```python
from build123d import *

# Parameters (mm, degrees)
SKETCH1_R           = 174.85
SKETCH1_R_2         = 3.556
SKETCH1_R_3         = 162.15
BOSS_EXTRUDE1_DEPTH = 3.175


with BuildPart() as part:
    # Sketch1 → Boss-Extrude1 (new body)
    with BuildSketch(Plane(origin=(0, 0, 0), x_dir=(1, 0, 0), z_dir=(0, 1, 0))):
        Circle(SKETCH1_R)
        with Locations((0, 168.5)):
            Circle(SKETCH1_R_2, mode=Mode.SUBTRACT)
        with Locations((145.925280538, 84.25)):
            Circle(SKETCH1_R_2, mode=Mode.SUBTRACT)
        with Locations((145.925280538, -84.25)):
            Circle(SKETCH1_R_2, mode=Mode.SUBTRACT)
        with Locations((0, -168.5)):
            Circle(SKETCH1_R_2, mode=Mode.SUBTRACT)
        with Locations((-145.925280538, -84.25)):
            Circle(SKETCH1_R_2, mode=Mode.SUBTRACT)
        with Locations((-145.925280538, 84.25)):
            Circle(SKETCH1_R_2, mode=Mode.SUBTRACT)
        Circle(SKETCH1_R_3, mode=Mode.SUBTRACT)
    extrude(amount=BOSS_EXTRUDE1_DEPTH)


solid = part.part
```
For this review, take the finished solid that the model builds, in its own axes (mm). Round coordinates to 2 decimals unless told otherwise and drop trailing zeros. Order: outer loops, then holes, each group sorted by start corner. A loop starts at its lowest first (then second) coordinate and runs counter-clockwise, first axis right, second up.
Q1. We need section C-C, the plane y = 2.35. Give the boundary of the cut face in (x, z).
Findings below:
outline: circle Ø349.7 at (0, 0); hole circle Ø324.3 at (0, 0); hole circle Ø7.11 at (-145.93, -84.25); hole circle Ø7.11 at (-145.93, 84.25); hole circle Ø7.11 at (0, -168.5); hole circle Ø7.11 at (0, 168.5); hole circle Ø7.11 at (145.93, -84.25); hole circle Ø7.11 at (145.93, 84.25)
Q2. Insertion check: P1, Ø1.5, axis at y = 2, z = 48.5, coming from the -X side. The pin has a flat end and moves straight along its axis. Give the tip position at first contact, or say it passes through.
Findings below:
P1: stops at x = -168.2
Q3. We need section A-A, the plane z = 0. Give the boundary of the cut face in (x, y) (3 decimals).
Findings below:
outline: (-174.85, 0) - (-162.15, 0) - (-162.15, 3.175) - (-174.85, 3.175) - close; (162.15, 0) - (174.85, 0) - (174.85, 3.175) - (162.15, 3.175) - close
Q4. We need section B-B, the plane x = -92. Give the boundary of the cut face in (y, z) (3 decimals).
Findings below:
outline: (0, -148.689) - (3.175, -148.689) - (3.175, -133.524) - (0, -133.524) - close; (0, 133.524) - (3.175, 133.524) - (3.175, 148.689) - (0, 148.689) - close
Q5. Wall thickness on line 1 (Z direction, x = 0, y = 2.1); line 2 (X direction, y = 1.1, z = 0); line 3 (Z direction, x = -3, y = 1.8): over which ranges is each line inside the solid? List them lowest first.
Findings below:
line 1: z = -174.85 to -172.06, -164.94 to -162.15, 162.15 to 164.94, 172.06 to 174.85
line 2: x = -174.85 to -162.15, 162.15 to 174.85
line 3: z = -174.82 to -170.41, -166.59 to -162.12, 162.12 to 166.59, 170.41 to 174.82
